```python
from build123d import *

# Parameters (mm, degrees)
SKETCH1_R           = 9.2075
BOSS_EXTRUDE1_DEPTH = 9.1694
BOSS_EXTRUDE1_TAPER = 2
SKETCH2_R           = 2.54
CUT_EXTRUDE1_DEPTH  = 23.491502958


with BuildPart() as part:
    # Sketch1 → Boss-Extrude1 (new body)
    with BuildSketch(Plane(origin=(0, 0, 0), x_dir=(1, 0, 0), z_dir=(0, 1, 0))):
        Circle(SKETCH1_R)
    boss_extrude1 = extrude(amount=BOSS_EXTRUDE1_DEPTH, taper=BOSS_EXTRUDE1_TAPER)

    # Mirror1: Boss-Extrude1 across plane
    add(boss_extrude1.mirror(Plane.ZX))

    # Sketch2 → Cut-Extrude1 (cut, through all)
    with BuildSketch(Plane(origin=(0, -9.1694, 0), x_dir=(-1, 0, 0), z_dir=(0, -1, 0))):
        with Locations(Location((0, 0, 0), (0, 0, 90))):
            Circle(SKETCH2_R)
    extrude(amount=-CUT_EXTRUDE1_DEPTH, mode=Mode.SUBTRACT)


solid = part.part
```
Work out the finished part from the listing and answer in its coordinate system (mm). Give positions to 0.01 mm unless a question says otherwise; leave off trailing zeros. Write each loop counter-clockwise with the first axis right and the second up, starting at its lowest first coordinate (ties: lowest second). Pieces come first, ordered by that corner, then holes. Notation, with made-up numbers: (-23, -38.75) -> (-4, -38.75) arc R10 ccw to (-4, -25.75) -> close; hole circle Ø6 at (46, 7.5). An arc over 180 degrees is marked (long way). Write item = value, one per line.
Q1. Section A-A on x = 0 is taken. Determine the outline of the cut face in (y, z), and give its area (3 significant figures).
Computed values:
outline = (-9.17, -8.89) -> (0, -9.21) -> (9.17, -8.89) -> (9.17, -2.54) -> (-9.17, -2.54) -> close; (-9.17, 2.54) -> (9.17, 2.54) -> (9.17, 8.89) -> (0, 9.21) -> (-9.17, 8.89) -> close
area = 239 mm^2
Q2. Flat-ended cylindrical pins translate along their axes: pin 1 Ø10 at (x, y) = (1, -0.5) entering from -Z; pin 2 Ø5 at (y, z) = (-6, 6) entering from -X; pin 3 Ø3 at (x, y) = (4.5, 6.5) entering from -Z; pin 4 Ø5 at (y, z) = (-7, 7.5) entering from -X. Find the tip coordinate at first contact, or state that the pin passes through.
Computed values:
pin_1 = -9.21
pin_2 = -8.29
pin_3 = -8.47
pin_4 = -7.44
Q3. Consider line 1 along Z through (x, y) = (1.75, 3); line 2 along X through (y, z) = (-1.25, 0); line 3 along X through (y, z) = (6.25, -2). Determine where each line is inside the solid, lowest interval first.
Computed values:
line_1 = -8.93 to -1.84, 1.84 to 8.93
line_2 = -9.16 to -2.54, 2.54 to 9.16
line_3 = -8.76 to -1.57, 1.57 to 8.76
Q4. Section B-B on y = 1.5 is taken. Determine the outline of the cut face in (x, z).
Computed values:
outline = circle Ø18.31 at (0, 0); hole circle Ø5.08 at (0, 0)
Q5. For a pull along Z with two mould halves and no side action, classify faces 1 (the conical face through (8.627, 4.649, -2.717)), 2 (the flat face through (2, 9.169, 2)), 3 (the cylindrical face through (2.52, -0.13, 0.33)) as pulls with the +Z half, pulls with the -Z half, needs draft (parallel to the pull), parting line crosses it, or undercut.
Computed values:
face_1 = parting line crosses it
face_2 = needs draft
face_3 = undercut
Q6. Section C-C on y = -4.25 is taken. Determine the outline of the cut face in (x, z).
Computed values:
outline = circle Ø18.12 at (0, 0); hole circle Ø5.08 at (0, 0)
